Geometry: final body of the model. Coordinates: model frame, mm. Face numbers are marked on the shaded views. A direction names the side the tool comes from. Give positions to 0.01 mm unless a question says otherwise; leave off trailing zeros. Write each loop counter-clockwise with the first axis right and the second up, starting at its lowest first coordinate (ties: lowest second). Pieces come first, ordered by that corner, then holes. Notation, with made-up numbers: M 43,60 L 47,60 A18 ccw 47,86 Z; hole C 84,33.5 d6. An arc over 180 degrees is marked long. Answer as a JSON object with one key per item and string values.
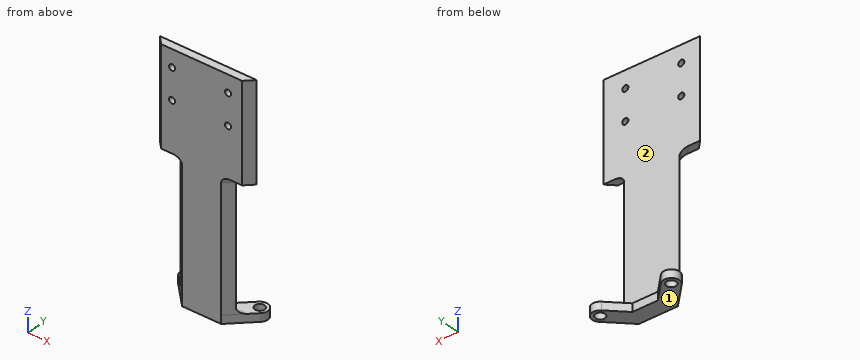
from build123d import *

# Parameters (mm, degrees)
BOSS_EXTRUDE1_DEPTH       = 3.175
SKETCH2_W                 = 15.330256122
SKETCH2_H                 = 3.175
BOSS_EXTRUDE2_DEPTH       = 50.8
FILLET1_R                 = 2.54
F_6_CLEARANCE_HOLE1_D     = 3.7973
F_6_CLEARANCE_HOLE1_DEPTH = 25.4
F_6_CLEARANCE_HOLE1_TIP   = 1.140824014
BOSS_EXTRUDE3_DEPTH       = 38.1
FILLET2_R                 = 2.54
M2_CLEARANCE_HOLE1_D      = 2.4
M2_CLEARANCE_HOLE1_DEPTH  = 25.4
M2_CLEARANCE_HOLE1_TIP    = 0.721032743


with BuildPart() as part:
    # Sketch1 → Boss-Extrude1 (new body)
    with BuildSketch(Plane.XY):
        with BuildLine():
            Line((-2.24506403, -2.24506403), (6.304871939, -10.795))
            Line((6.304871939, -10.795), (21.635128061, -10.795))
            Line((21.635128061, -10.795), (30.18506403, -2.24506403))
            ThreePointArc((30.18506403, -2.24506403), (30.18506403, 2.24506403), (25.69493597, 2.24506403))
            Line((25.69493597, 2.24506403), (19.004871939, -4.445))
            Line((19.004871939, -4.445), (8.935128061, -4.445))
            Line((8.935128061, -4.445), (2.24506403, 2.24506403))
            ThreePointArc((2.24506403, 2.24506403), (-2.24506403, 2.24506403), (-2.24506403, -2.24506403))
        make_face()
    extrude(amount=BOSS_EXTRUDE1_DEPTH)

    # Sketch2 → Boss-Extrude2 (add)
    with BuildSketch(Plane.XY.offset(3.175)):
        with Locations((13.97, -9.2075)):
            Rectangle(SKETCH2_W, SKETCH2_H)
        Polygon((3.129871939, -7.62), (6.304871939, -10.795), (6.304871939, -7.62), align=None)
        Polygon((21.635128061, -7.62), (21.635128061, -10.795), (24.810128061, -7.62), align=None)
    extrude(amount=BOSS_EXTRUDE2_DEPTH)

    # Fillet1
    fillet1_edges = [part.edges().sort_by_distance(p)[0] for p in [
        (13.97, -7.62, 3.175),
    ]]
    fillet(fillet1_edges, radius=FILLET1_R)

    # #6 Clearance Hole1
    with Locations(Plane(origin=(0, 0, 0), x_dir=(-1, 0, 0), z_dir=(0, 0, -1))):
        with Locations((-27.94, 0), (0, 0)):
            Hole(F_6_CLEARANCE_HOLE1_D / 2, depth=F_6_CLEARANCE_HOLE1_DEPTH)
            with Locations((0, 0, -(F_6_CLEARANCE_HOLE1_DEPTH + F_6_CLEARANCE_HOLE1_TIP / 2))):  # 118° drill point
                Cone(0, F_6_CLEARANCE_HOLE1_D / 2, F_6_CLEARANCE_HOLE1_TIP, mode=Mode.SUBTRACT)

    # Sketch7 → Boss-Extrude3 (add)
    with BuildSketch(Plane.XY.offset(53.975)):
        Polygon((-5.080004961, -7.62), (33.019995039, -7.62), (29.844995039, -10.795), (-1.905004961, -10.795), align=None)
    extrude(amount=BOSS_EXTRUDE3_DEPTH)

    # Fillet2
    fillet2_edges = [part.edges().sort_by_distance(p)[0] for p in [
        (4.717371939, -9.2075, 53.975),
        (23.222628061, -9.2075, 53.975),
    ]]
    fillet(fillet2_edges, radius=FILLET2_R)

    # M2 Clearance Hole1
    with Locations(Plane(origin=(0, -7.62, 0), x_dir=(-1, 0, 0), z_dir=(0, 1, 0))):
        with Locations((-2.354305281, 85.375), (-2.354305281, 73.375), (-24.354305281, 85.375), (-24.354305281, 73.375)):
            Hole(M2_CLEARANCE_HOLE1_D / 2, depth=M2_CLEARANCE_HOLE1_DEPTH)
            with Locations((0, 0, -(M2_CLEARANCE_HOLE1_DEPTH + M2_CLEARANCE_HOLE1_TIP / 2))):  # 118° drill point
                Cone(0, M2_CLEARANCE_HOLE1_D / 2, M2_CLEARANCE_HOLE1_TIP, mode=Mode.SUBTRACT)


solid = part.part
1) Set-up query: the marked faces 1 and 2. Return all of +Z, -Z, +X, -X, +Y, -Y with unobstructed straight access to the full face (end or side cutting, diameter ignored); none if empty.
Geometry check:
{"face 1": "-Z, +X, -X, +Y, -Y", "face 2": "+Z, +X, -X, +Y"}
2) Cut plane D-D on y = -9.25. Give the number of separate pieces and of enclosed holes in the cut face, and give its area (3 significant figures).
Geometry check:
{"separate pieces": "1", "enclosed holes": "4", "area": "2,310 mm2"}
3) Cut plane B-B on y = 0. Return loops of the section in (x, z) (3 decimals), and give its area (3 significant figures).
Geometry check:
{"outline": "M -3.175,0 L -1.899,0 L -1.899,3.175 L -3.175,3.175 Z; M 1.899,0 L 4.49,0 L 4.49,3.175 L 1.899,3.175 Z; M 23.45,0 L 26.041,0 L 26.041,3.175 L 23.45,3.175 Z; M 29.839,0 L 31.115,0 L 31.115,3.175 L 29.839,3.175 Z", "area": "24.6 mm2"}
4) Contact query for flat-ended pins moving along their axis: P1, Ø2.5, axis at x = 14, z = 2, coming from the +Y side (3 decimals); P2, Ø4, axis at x = 2.35, z = 73.38, coming from the +Y side; P3, Ø5, axis at x = 27.94, y = 0, coming from the +Z side (3 decimals). Output: stop coordinate, or through.
Geometry check:
{"P1": "stops at y = -4.445", "P2": "stops at y = -7.62", "P3": "stops at z = 3.175"}
5) Cut plane C-C on z = 70. Return loops of the section in (x, y) (3 decimals).
Geometry check:
{"outline": "M -5.08,-7.62 L -1.905,-10.795 L 29.845,-10.795 L 33.02,-7.62 Z"}
6) Cut plane A-A on x = 17. Return loops of the section in (y, z) (3 decimals).
Geometry check:
{"outline": "M -10.795,0 L -4.445,0 L -4.445,3.175 L -5.08,3.175 A2.54 cw -7.62,5.715 L -7.62,92.075 L -10.795,92.075 Z"}
7) Line query: line 1 (Y direction, x = 11.5, z = 53) (3 decimals); line 2 (Z direction, x = -2, y = -9.25) (3 decimals); line 3 (Y direction, x = 23.5, z = 11). Output: solid intervals per line, ascending. Write a range as from..to.
Geometry check:
{"line 1": "y = -10.795..-7.62", "line 2": "z = 53.975..92.075", "line 3": "y = -8.93..-7.62"}
